Autodesk Inventor part; units mm, degrees
ref_plane "YZ Plane" through (0, 0, 0) normal (1, 0, 0) x (0, 1, 0)
ref_plane "XZ Plane" through (0, 0, 0) normal (0, 1, 0) x (-1, 0, 0)
ref_plane "XY Plane" through (0, 0, 0) normal (0, 0, 1) x (1, 0, 0)
sketch "Sketch1" plane through (0, 0, 0) normal (0, 0, 1) x (1, 0, 0)
  line L0 (0, 0) -> (300, 0)
  line L1 (300, 0) -> (300, 200)
  line L2 (300, 200) -> (0, 200)
  line L3 (0, 200) -> (0, 0)
  line L4 (10, 10) -> (290, 10)
  line L5 (290, 10) -> (290, 190)
  line L6 (290, 190) -> (10, 190)
  line L7 (10, 190) -> (10, 10)
  line L8 (13.75, 13.75) -> (286.25, 13.75)
  line L9 (286.25, 13.75) -> (286.25, 186.25)
  line L10 (286.25, 186.25) -> (13.75, 186.25)
  line L11 (13.75, 186.25) -> (13.75, 13.75)
  line L12 (38.75, 190) -> (68.5, 190)
  line L13 (68.5, 190) -> (68.5, 186.25)
  line L14 (68.5, 186.25) -> (38.75, 186.25)
  line L15 (38.75, 186.25) -> (38.75, 190)
  line L16 (10, 161.25) -> (13.75, 161.25)
  line L17 (13.75, 161.25) -> (13.75, 131.5)
  line L18 (13.75, 131.5) -> (10, 131.5)
  line L19 (10, 131.5) -> (10, 161.25)
  line L20 (0, 0) -> (150, 0)
  line L21 (150, 0) -> (150, 100)
  line L22 (150, 100) -> (0, 100)
  line L23 (0, 100) -> (0, 0)
  line L24 (38.75, 10) -> (68.5, 10)
  line L25 (68.5, 10) -> (68.5, 13.75)
  line L26 (68.5, 13.75) -> (38.75, 13.75)
  line L27 (38.75, 13.75) -> (38.75, 10)
  line L28 (10, 38.75) -> (13.75, 38.75)
  line L29 (13.75, 38.75) -> (13.75, 68.5)
  line L30 (13.75, 68.5) -> (10, 68.5)
  line L31 (10, 68.5) -> (10, 38.75)
  line L32 (150, 200) -> (150, 100)
  line L33 (300, 200) -> (300, 0)
  line L34 (261.25, 190) -> (231.5, 190)
  line L35 (231.5, 190) -> (231.5, 186.25)
  line L36 (231.5, 186.25) -> (261.25, 186.25)
  line L37 (261.25, 186.25) -> (261.25, 190)
  line L38 (290, 161.25) -> (286.25, 161.25)
  line L39 (286.25, 161.25) -> (286.25, 131.5)
  line L40 (286.25, 131.5) -> (290, 131.5)
  line L41 (290, 131.5) -> (290, 161.25)
  line L42 (300, 100) -> (300, 0)
  line L43 (261.25, 13.75) -> (261.25, 10)
  line L44 (231.5, 10) -> (231.5, 13.75)
  line L45 (231.5, 13.75) -> (261.25, 13.75)
  line L46 (261.25, 10) -> (231.5, 10)
  line L47 (286.25, 68.5) -> (290, 68.5)
  line L48 (290, 38.75) -> (286.25, 38.75)
  line L49 (290, 68.5) -> (290, 38.75)
  line L50 (286.25, 38.75) -> (286.25, 68.5)
  point P0 (13.75, 161.25)
  point P1 (10, 131.5)
  point P2 (10, 68.5)
  point P3 (13.75, 68.5)
  point P4 (13.75, 38.75)
  point P5 (10, 38.75)
  point P6 (68.5, 13.75)
  point P7 (68.5, 10)
  point P8 (38.75, 10)
  point P9 (38.75, 13.75)
  point P10 (231.5, 186.25)
  point P11 (231.5, 190)
  point P12 (261.25, 190)
  point P13 (261.25, 186.25)
  point P14 (286.25, 131.5)
  point P15 (286.25, 161.25)
  point P16 (290, 161.25)
  point P17 (261.25, 13.75)
  point P18 (261.25, 10)
  point P19 (231.5, 10)
  point P20 (231.5, 13.75)
  point P21 (286.25, 68.5)
  point P22 (286.25, 38.75)
  point P23 (68.5, 190)
  dimension "d0" = 300
  dimension "d1" = 200
  dimension "d2" = 280
  dimension "d3" = 180
  dimension "d4" = 10
  dimension "d5" = 10
  dimension "d6" = 3.75
  dimension "d7" = 3.75
  dimension "d8" = 3.75
  dimension "d9" = 3.75
  dimension "d10" = 25
  dimension "d11" = 29.75
  dimension "d12" = 29.75
  dimension "d13" = 25
  dimension "d14" = 100
  dimension "d15" = 150
extrude "Extrusion1" add sketch "Sketch1" along normal blind 4 contours L3 L22 L7 L4 L21 L0 | L21 L4 L5 L6 L32 L2 L1 L0 | L3 L2 L32 L6 L7 L22 | L21 L8 L44 L4 | L4 L25 L8 L21 | L22 L11 L30 L7 | L7 L18 L11 L22 | L21 L32 L10 L9 L8 | L8 L11 L22 L21 | L11 L10 L32 L22 | L4 L7 L28 L11 L8 L27 | L43 L8 L9 L48 L5 L4 | L32 L10 L13 L6 | L6 L35 L10 L32 | L7 L6 L15 L10 L11 L16 | L6 L5 L38 L9 L10 L37 | L47 L9 L40 L5
sketch "Sketch5" plane through (0, 0, 4) normal (0, 0, 1) x (1, 0, 0)
  line L0 (103.75, 114.875) -> (107.5, 114.875)
  line L1 (107.5, 114.875) -> (107.5, 85.125)
  line L2 (107.5, 85.125) -> (103.75, 85.125)
  line L3 (103.75, 85.125) -> (103.75, 114.875)
  line L4 (13.75, 68.5) -> (13.75, 38.75)
  line L5 (0, 0) -> (300, 0)
  point P0 (107.5, 100)
  dimension "d53" = 3.75
  dimension "d54" = 29.75
  dimension "d55" = 90
  dimension "d56" = 100
extrude "Extrusion5" cut sketch "Sketch5" against normal through all
sketch "Sketch6" plane through (0, 0, 0) normal (0, 0, -1) x (-1, 0, 0)
  circle A0 centre (-258.8334, 28.75) radius 1.5
  circle A1 centre (-143.8334, 28.75) radius 1.5
  circle A2 centre (-143.8334, 103.75) radius 1.5
  line L0 (-300, 0) -> (-300, 200)
  line L1 (-231.5, 13.75) -> (-261.25, 13.75)
  circle A3 centre (-196.25, 171.25) radius 3
  circle A4 centre (-196.25, 131.25) radius 3
  line L2 (-286.25, 131.5) -> (-286.25, 161.25)
  line L3 (-261.25, 186.25) -> (-231.5, 186.25)
  point P0 (0, 0)
  dimension "d59" = 41.1666
  dimension "d60" = 115
  dimension "d61" = 75
  dimension "d62" = 0
  dimension "d63" = 3
  dimension "d64" = 3
  dimension "d65" = 3
  dimension "d66" = 15
  dimension "d67" = 15
  dimension "d70" = 40
  dimension "d71" = 6
  dimension "d72" = 6
  dimension "d73" = 90
  dimension "d74" = 90
  dimension "d75" = 15
extrude "Extrusion6" cut sketch "Sketch6" against normal through all
sketch "Sketch7" plane through (0, 0, 0) normal (0, 0, -1) x (-1, 0, 0)
  line L0 (-290, 146.5) -> (-286.25, 146.5)
  line L1 (-286.25, 146.5) -> (-286.25, 86.5)
  line L2 (-286.25, 86.5) -> (-290, 86.5)
  line L3 (-290, 86.5) -> (-290, 146.5)
  line L4 (-290, 161.25) -> (-290, 131.5)
  line L5 (-286.25, 131.5) -> (-286.25, 161.25)
  line L6 (-290, 131.5) -> (-286.25, 131.5)
  line L7 (-290, 68.5) -> (-290, 38.75)
  line L8 (-286.25, 38.75) -> (-286.25, 68.5)
  line L9 (-290, 68.5) -> (-286.25, 68.5)
  line L10 (-286.25, 68.5) -> (-286.25, 38.75)
  line L11 (-286.25, 38.75) -> (-290, 38.75)
  line L12 (-290, 38.75) -> (-290, 68.5)
  line L13 (-290, 161.25) -> (-290, 131.5)
  line L14 (-290, 161.25) -> (-286.25, 161.25)
  line L15 (-286.25, 161.25) -> (-286.25, 146.5)
  line L16 (-286.25, 146.5) -> (-290, 146.5)
  line L17 (-290, 146.5) -> (-290, 161.25)
  point P0 (0, 0)
  dimension "d79" = 0
  dimension "d80" = 0
  dimension "d81" = 15
  dimension "d82" = 60
extrude "Extrusion7" add sketch "Sketch7" against normal blind 4 contours L4 L14 L5 L0 | L9 L8 L11 L7
extrude "Extrusion8" cut sketch "Sketch7" against normal through all contours L0 L1 L6 L3 | L6 L1 L2 L3
sketch "Sketch8" plane through (0, 0, 0) normal (0, 0, -1) x (-1, 0, 0)
  line L0 (-261.25, 190) -> (-261.25, 186.25)
  line L1 (-261.25, 190) -> (-201.25, 190)
  line L2 (-201.25, 190) -> (-201.25, 186.25)
  line L3 (-201.25, 186.25) -> (-261.25, 186.25)
  line L4 (-261.25, 186.25) -> (-261.25, 190)
  line L5 (-261.25, 13.75) -> (-261.25, 10)
  line L6 (-261.25, 13.75) -> (-201.25, 13.75)
  line L7 (-201.25, 13.75) -> (-201.25, 10)
  line L8 (-201.25, 10) -> (-261.25, 10)
  line L9 (-261.25, 10) -> (-261.25, 13.75)
  point P0 (0, 0)
  dimension "d87" = 60
  dimension "d88" = 3.75
  dimension "d89" = 3.75
extrude "Extrusion9" cut sketch "Sketch8" against normal through all
properties part number "onderstuk_8AUG"
Input: part model. Units: mm. Frame: model coordinates. Round coordinates to 2 decimals unless told otherwise and drop trailing zeros. Write each loop counter-clockwise with the first axis right and the second up, starting at its lowest first coordinate (ties: lowest second). Pieces come first, ordered by that corner, then holes.
1) Cut plane C-C (z = 1). Count the separate pieces of the cut face and the enclosed holes in it, then the cut area to 3 significant figures.
2) Cut plane B-B (y = 140). Return the cut outline in (x, z).
3) Ray query, L1, parallel to X at y = 103.75, z = 1.3; L2, parallel to Y at x = 229, z = 0.8; L3, parallel to X at y = 112, z = 2.65. Return the intervals inside material, ascending.
4) Draft query along X for faces 1 (the flat face through (148, 101, 0)), 2 (the cylindrical face through (194.64, 173.78, 1.97)). Return one class per face: pulls with the +X half, pulls with the -X half, needs draft (parallel to the pull), parting line crosses it, or undercut.
5) Cut plane A-A (x = 227). Return the cut outline in (y, z).
Geometry says:
1. separate pieces: 1
1. enclosed holes: 13
1. area: 58,700 mm2
2. outline: (0, 0) - (10, 0) - (10, 4) - (0, 4) - close; (13.75, 0) - (286.25, 0) - (286.25, 4) - (13.75, 4) - close; (290, 0) - (300, 0) - (300, 4) - (290, 4) - close
3. L1: x = 0 to 103.75, 107.5 to 142.33, 145.33 to 286.25, 290 to 300
3. L2: y = 0 to 10, 13.75 to 186.25, 190 to 200
3. L3: x = 0 to 103.75, 107.5 to 286.25, 290 to 300
4. face 1: needs draft
4. face 2: undercut
5. outline: (0, 0) - (10, 0) - (10, 4) - (0, 4) - close; (13.75, 0) - (186.25, 0) - (186.25, 4) - (13.75, 4) - close; (190, 0) - (200, 0) - (200, 4) - (190, 4) - close
